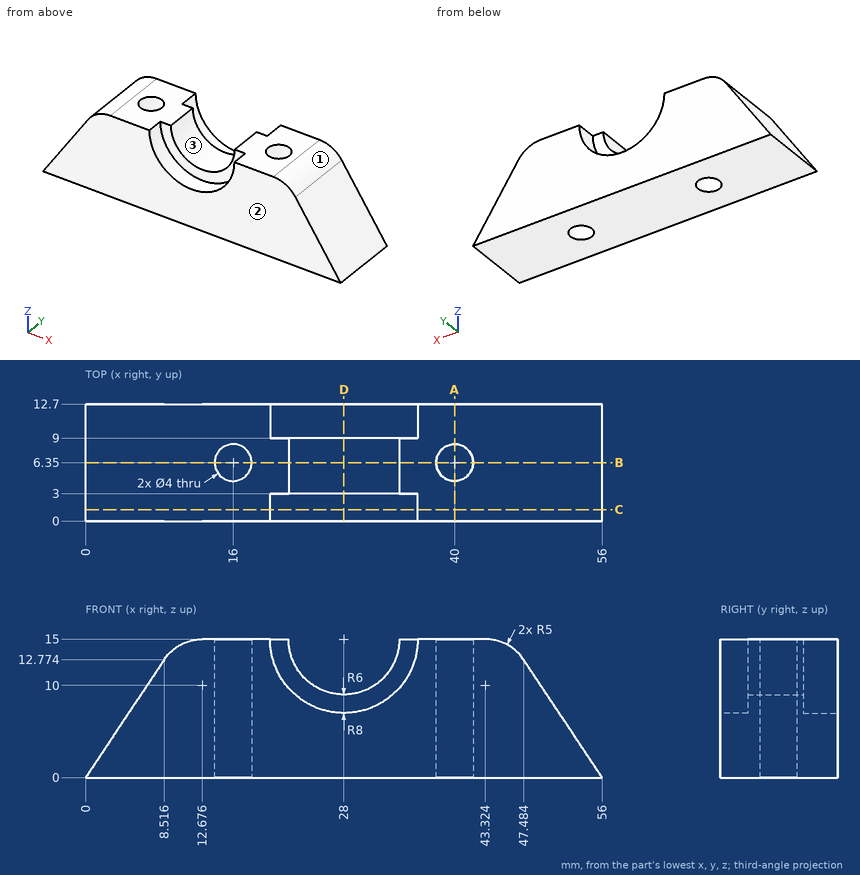
Input: dimensioned drawing with shaded views. Units: mm. Origin: part minimum x, y, z. Round coordinates to 2 decimals unless told otherwise and drop trailing zeros. Loops run counter-clockwise (first coordinate to the right, second up) from the corner with the lowest first, then second, coordinate; pieces in that order, holes last. Notation, with made-up numbers: M 56,-15 L 82,-15 A21 ccw 82,-8 Z; hole C 16,15.5 d3. An arc over 180 degrees is marked long. Return JSON: item names as keys, results as strings. Group by question number.
1. Section query B-B on y = 6.35. Output: boundary loops of the cut face in (x, z) (1 decimal).
2. Mould query, pull axis X, two halves, no side actions, for the marked faces 1, 2 and 3. Classes: released by +X, released by -X, zero draft, split by the parting line, or undercut.
3. Section query C-C on y = 1.25. Output: boundary loops of the cut face in (x, z) (1 decimal), and give its area (3 significant figures).
4. Pin query (flat end, axial travel): pin 1 (6 mm diameter, centred on x = 27, y = 2.5, fed in from +Z); pin 2 (1.5 mm diameter, centred on y = 10.5, z = 11.5, fed in from -X); pin 3 (4 mm diameter, centred on y = 1.5, z = 7, fed in from +X). Return the tip coordinate at first contact, or that it passes through.
5. Material intervals for line 1 along Y through (x, z) = (16, 4.25); line 2 along X through (y, z) = (6.5, 10.25) (1 decimal); line 3 along X through (y, z) = (5.5, 5.25), sorted ascending. Write a range as from..to.
6. Section query A-A on x = 40. Output: boundary loops of the cut face in (y, z).
7. Section query D-D on x = 28. Output: boundary loops of the cut face in (y, z).
Checks:
{
 "1": {"outline": "M 0,0 L 14,0 L 14,15 L 12.7,15 A5 ccw 8.5,12.8 Z; M 18,0 L 38,0 L 38,15 L 34,15 A6 cw 22,15 L 18,15 Z; M 42,0 L 56,0 L 47.5,12.8 A5 ccw 43.3,15 L 42,15 Z"},
 "2": {"face 1": "released by +X", "face 2": "zero draft", "face 3": "undercut"},
 "3": {"outline": "M 0,0 L 56,0 L 47.5,12.8 A5 ccw 43.3,15 L 36,15 A8 cw 20,15 L 12.7,15 A5 ccw 8.5,12.8 Z", "area": "587 mm²"},
 "4": {"pin 1": "stops at z = 10.49", "pin 2": "stops at x = 7.17", "pin 3": "stops at x = 52.67"},
 "5": {"line 1": "y = 0..4.35, 8.35..12.7", "line 2": "x = 6.8..14, 18..24.3, 31.7..38, 42..49.2", "line 3": "x = 3.5..14.19, 17.81..38.19, 41.81..52.5"},
 "6": {"outline": "M 0,0 L 4.35,0 L 4.35,15 L 0,15 Z; M 8.35,0 L 12.7,0 L 12.7,15 L 8.35,15 Z"},
 "7": {"outline": "M 0,0 L 12.7,0 L 12.7,7 L 9,7 L 9,9 L 3,9 L 3,7 L 0,7 Z"}
}
